Source: CAD feature listing. Evaluate the final solid. Frame: model axes, mm. A direction names the side the tool comes from. Give positions to 0.01 mm unless a question says otherwise; leave off trailing zeros. Write each loop counter-clockwise with the first axis right and the second up, starting at its lowest first coordinate (ties: lowest second). Pieces come first, ordered by that corner, then holes. Notation, with made-up numbers: (29, 48) -> (57, 48) arc R34 ccw to (57, 82) -> close; hole circle Ø6 at (-7.5, -12). An arc over 180 degrees is marked (long way). Write item = value, one per line.
from build123d import *

# Parameters (mm, degrees)
SKETCH1_R                      = 5
EXTRUDE1_DEPTH                 = 4
CIRPATTERN2_COUNT              = 3
EXTRUDE4_START                 = 4.45086
EXTRUDE4_DEPTH                 = 7.205259
EXTRUDE5_START                 = 4.330127
EXTRUDE5_DEPTH                 = 7.205258
EXTRUDE6_START                 = 4.330127
EXTRUDE6_DEPTH                 = 7.205258
SKETCH11_W                     = 14.943105969
SKETCH11_H                     = 2.182700872
EXTRUDE7_DEPTH                 = 10
F_0_5_0_5_DIAMETER_HOLE1_D     = 0.5
F_0_5_0_5_DIAMETER_HOLE1_DEPTH = 0.25
F_0_5_0_5_DIAMETER_HOLE1_TIP   = 0.150215155
F_0_5_0_5_DIAMETER_HOLE2_D     = 0.5
F_0_5_0_5_DIAMETER_HOLE2_DEPTH = 0.25
F_0_5_0_5_DIAMETER_HOLE2_TIP   = 0.150215155
F_0_5_0_5_DIAMETER_HOLE3_D     = 0.5
F_0_5_0_5_DIAMETER_HOLE3_DEPTH = 0.25
F_0_5_0_5_DIAMETER_HOLE3_TIP   = 0.150215155


with BuildPart() as part:
    # Sketch1 → Extrude1 (new body)
    with BuildSketch(Plane(origin=(0, 0, 0), x_dir=(1, 0, 0), z_dir=(0, 1, 0))):
        with BuildLine():
            Line((-9.989936491, 3.146959138), (-8.459547932, 0.4962484))
            ThreePointArc((-8.459547932, 0.4962484), (-8.203164753, -0.718531203), (-8.713035455, -1.850544314))
            ThreePointArc((-8.713035455, -1.850544314), (-9.09326674, -5.370733384), (-5.854577936, -6.801537968))
            ThreePointArc((-5.854577936, -6.801537968), (-4.619290473, -6.925983542), (-3.695452068, -7.75540769))
            Line((-3.695452068, -7.75540769), (-2.165063509, -10.406118428))
            ThreePointArc((-2.165063509, -10.406118428), (0, -11.656118428), (2.165063509, -10.406118428))
            Line((2.165063509, -10.406118428), (3.695452068, -7.75540769))
            ThreePointArc((3.695452068, -7.75540769), (4.619290473, -6.925983542), (5.854577936, -6.801537968))
            ThreePointArc((5.854577936, -6.801537968), (9.09326674, -5.370733384), (8.713035455, -1.850544314))
            ThreePointArc((8.713035455, -1.850544314), (8.203164753, -0.718531203), (8.459547932, 0.4962484))
            Line((8.459547932, 0.4962484), (9.989936491, 3.146959138))
            ThreePointArc((9.989936491, 3.146959138), (9.989936491, 5.646959138), (7.824872981, 6.896959138))
            Line((7.824872981, 6.896959138), (4.764095865, 6.896959138))
            ThreePointArc((4.764095865, 6.896959138), (3.583874279, 7.282314592), (2.858457519, 8.289882129))
            ThreePointArc((2.858457519, 8.289882129), (0, 10.379266616), (-2.858457519, 8.289882129))
            ThreePointArc((-2.858457519, 8.289882129), (-3.583874279, 7.282314592), (-4.764095865, 6.896959138))
            Line((-4.764095865, 6.896959138), (-7.824872981, 6.896959138))
            ThreePointArc((-7.824872981, 6.896959138), (-9.989936491, 5.646959138), (-9.989936491, 3.146959138))
        make_face()
        with Locations((0, -0.120733384)):
            Circle(SKETCH1_R, mode=Mode.SUBTRACT)
    extrude(amount=EXTRUDE1_DEPTH)

    # Sketch6 → M3 Clearance Hole1 (revolve, cut)
    with BuildSketch(Plane(origin=(-6.495190528, 4, 3.870733384), x_dir=(0, 0, 1), z_dir=(1, 0, 0))):
        Polygon((0, 0), (0, 11.021463052), (1.7, 10), (1.7, 0), align=None)
    m3_clearance_hole1 = revolve(axis=Axis((-6.495190528, 10.35, 3.870733384), (0, -1, 0)), mode=Mode.SUBTRACT)

    # CirPattern2: M3 Clearance Hole1 ×3 about axis
    cirpattern2_axis = Axis((0, 0, 0.120733384), (0, 1, 0))
    for i in range(1, CIRPATTERN2_COUNT):
        add(m3_clearance_hole1.rotate(cirpattern2_axis, i * 360 / CIRPATTERN2_COUNT), mode=Mode.SUBTRACT)

    # GrooveSketch → Extrude4 (cut)
    with BuildSketch(Plane.XY.offset(EXTRUDE4_START)):
        Polygon((28.569876563, -26.069876563), (2.5, 0), (0, 2.5), (-2.5, 0), (-28.569876563, -26.069876563), (-28.569876563, -99.806622573), (28.569876563, -99.806622573), align=None)
    extrude(amount=EXTRUDE4_DEPTH, mode=Mode.SUBTRACT)

    # Sketch9 → Extrude5 (cut)
    with BuildSketch(Plane(origin=(0.052279089, 0, 0.030183346), x_dir=(-0.5, 0, 0.866025404), z_dir=(-0.866025404, 0, -0.5)).offset(EXTRUDE5_START)):
        Polygon((35.272745822, -32.668187644), (2.604558178, 0), (0.104558178, 2.5), (-2.395441822, 0), (-35.063629467, -32.668187644), (-35.063629467, -125.067775694), (35.272745822, -125.067775694), align=None)
    extrude(amount=EXTRUDE5_DEPTH, mode=Mode.SUBTRACT)

    # Sketch10 → Extrude6 (cut)
    with BuildSketch(Plane(origin=(-0.052279089, 0, 0.030183346), x_dir=(-0.5, 0, -0.866025404), z_dir=(0.866025404, 0, -0.5)).offset(EXTRUDE6_START)):
        Polygon((35.063629467, -32.668187644), (2.395441822, 0), (-0.104558178, 2.5), (-2.604558178, 0), (-35.272745822, -32.668187644), (-35.272745822, -125.067775694), (35.063629467, -125.067775694), align=None)
    extrude(amount=EXTRUDE6_DEPTH, mode=Mode.SUBTRACT)

    # Sketch11 → Extrude7 (cut)
    with BuildSketch(Plane(origin=(0, 4, 0), x_dir=(-1, 0, 0), z_dir=(0, 1, 0))):
        with Locations((-0.195883412, -10.988309574)):
            Rectangle(SKETCH11_W, SKETCH11_H)
    extrude(amount=-EXTRUDE7_DEPTH, mode=Mode.SUBTRACT)

    # Ø0.5 (0.5) Diameter Hole1
    with Locations(Plane(origin=(0, 2.5, -9.896959138), x_dir=(-1, 0, 0), z_dir=(0, 0, -1))):
        with Locations((0, 0)):
            Hole(F_0_5_0_5_DIAMETER_HOLE1_D / 2, depth=F_0_5_0_5_DIAMETER_HOLE1_DEPTH)
            with Locations((0, 0, -(F_0_5_0_5_DIAMETER_HOLE1_DEPTH + F_0_5_0_5_DIAMETER_HOLE1_TIP / 2))):  # 118° drill point
                Cone(0, F_0_5_0_5_DIAMETER_HOLE1_D / 2, F_0_5_0_5_DIAMETER_HOLE1_TIP, mode=Mode.SUBTRACT)

    # Ø0.5 (0.5) Diameter Hole2
    with Locations(Plane(origin=(6.5, 2.5, -6.896959138), x_dir=(-1, 0, 0), z_dir=(0, 0, -1))):
        with Locations((0, 0)):
            Hole(F_0_5_0_5_DIAMETER_HOLE2_D / 2, depth=F_0_5_0_5_DIAMETER_HOLE2_DEPTH)
            with Locations((0, 0, -(F_0_5_0_5_DIAMETER_HOLE2_DEPTH + F_0_5_0_5_DIAMETER_HOLE2_TIP / 2))):  # 118° drill point
                Cone(0, F_0_5_0_5_DIAMETER_HOLE2_D / 2, F_0_5_0_5_DIAMETER_HOLE2_TIP, mode=Mode.SUBTRACT)

    # Ø0.5 (0.5) Diameter Hole3
    with Locations(Plane(origin=(-6.5, 2.5, -6.896959138), x_dir=(-1, 0, 0), z_dir=(0, 0, -1))):
        with Locations((0, 0)):
            Hole(F_0_5_0_5_DIAMETER_HOLE3_D / 2, depth=F_0_5_0_5_DIAMETER_HOLE3_DEPTH)
            with Locations((0, 0, -(F_0_5_0_5_DIAMETER_HOLE3_DEPTH + F_0_5_0_5_DIAMETER_HOLE3_TIP / 2))):  # 118° drill point
                Cone(0, F_0_5_0_5_DIAMETER_HOLE3_D / 2, F_0_5_0_5_DIAMETER_HOLE3_TIP, mode=Mode.SUBTRACT)


solid = part.part
(1) Section query B-B (x = 1.25). Return loops of the section in (y, z).
Values follow:
outline = (0, -9.9) -> (4, -9.9) -> (4, -8.53) -> (0, -8.53) -> close; (0, -6.23) -> (4, -6.23) -> (4, -4.72) -> (0, -4.72) -> close; (1.25, 4.96) -> (4, 4.96) -> (4, 11.32) -> (1.25, 11.32) -> close
(2) Pull-direction query (X, two-part tool) for faces 5 (the face through (4.603, 1.972, 6.933)), 6 (the face through (-3.57, 1.972, -7.293)), 7 (the face through (1.5, 0, -5.8)); classes: pulls with the +X half, pulls with the -X half, needs draft (parallel to the pull), parting line crosses it, or undercut.
Values follow:
face_5 = undercut
face_6 = pulls with the -X half
face_7 = needs draft
(3) Section query A-A (z = -3.75). Return loops of the section in (x, y).
Values follow:
outline = (-10.24, 0.73) -> (-6.7, 2.5) -> (-3.17, 0.73) -> (-3.17, 4) -> (-10.24, 4) -> close; (3.17, 0.73) -> (6.7, 2.5) -> (10.24, 0.73) -> (10.24, 4) -> (3.17, 4) -> close
(4) Access query for faces 1 (the face through (6, 2, -6.897)), 2 (the face through (6.19, 1.23, -4.92)), 3 (the face through (-6, 2, -6.897)), 4 (the face through (1.3, 1.2, 8)). Directions: +Z, -Z, +X, -X, +Y, -Y. A direction counts if a zero-diameter tool reaches every point of the face in a straight line with its end or side. Return the directions, or none.
Values follow:
face_1 = -Z, +X, +Y, -Y
face_2 = -Y
face_3 = -Z, -X, +Y, -Y
face_4 = +Z, -Y
(5) Section query D-D (z = 8). Return loops of the section in (x, y), plus the area to 3 significant figures.
Values follow:
outline = (-3.55, 0) -> (-2.5, 0) -> (0, 2.5) -> (2.5, 0) -> (3.55, 0) -> (3.55, 4) -> (-3.55, 4) -> close
area = 22.2 mm2
(6) Section query C-C (y = 1.15). Give the number of separate pieces and of enclosed holes in the cut face, plus the area to 3 significant figures.
Values follow:
separate_pieces = 3
enclosed_holes = 3
area = 138 mm2
(7) Material intervals for line 1 (Y direction, x = 0, z = -9.75); line 2 (Z direction, x = 6, y = 2.2); line 3 (X direction, y = 2.5, z = -6.7), sorted ascending.
Values follow:
line_1 = 0 to 2.25, 2.75 to 4
line_2 = -6.9 to -3.69, -3 to 2.24, 5.5 to 6.83
line_3 = -8.8 to -6.75, -6.25 to -1.56, 1.56 to 6.25, 6.75 to 8.8
(8) First-contact query: pin 1 (5.5 mm diameter, centred on x = 0, z = -7.38, fed in from -Y); pin 2 (0.9 mm diameter, centred on x = 7, y = 1, fed in from -Z); pin 3 (6 mm diameter, centred on x = 0, z = 0.12, fed in from +Y); pin 4 (1.5 mm diameter, centred on y = 1, z = 8.5, fed in from +X). Flat tips, straight axial feed; report the tip coordinate or a pass-through.
Values follow:
pin_1 = 0
pin_2 = -6.9
pin_3 = through
pin_4 = 3.7
